```python
from build123d import *

# Parameters (mm, degrees)
SKETCH1_R           = 9
BOSS_EXTRUDE1_DEPTH = 27
BOSS_EXTRUDE2_DEPTH = 11.5


with BuildPart() as part:
    # Sketch1 → Boss-Extrude1 (new body, symmetric)
    with BuildSketch(Plane.XY):
        Circle(SKETCH1_R)
    extrude(amount=BOSS_EXTRUDE1_DEPTH, both=True)

    # Sketch2 → Boss-Extrude2 (add, symmetric)
    with BuildSketch(Plane.XY):
        with BuildLine():
            ThreePointArc((1.592403849, 11.893874473), (0, 12), (-1.592403849, 11.893874473))
            ThreePointArc((-1.592403849, 11.893874473), (-2.170910027, 15.684139908), (-4.926417678, 18.350215499))
            ThreePointArc((-4.926417678, 18.350215499), (-5.35291858, 18.230366499), (-5.776509232, 18.100606097))
            ThreePointArc((-5.776509232, 18.100606097), (-6.653200491, 14.368020679), (-5.090698654, 10.866682438))
            ThreePointArc((-5.090698654, 10.866682438), (-6.487689809, 10.095042394), (-7.769929381, 9.144845401))
            ThreePointArc((-7.769929381, 9.144845401), (-10.305771951, 12.020655535), (-14.065241784, 12.773761136))
            ThreePointArc((-14.065241784, 12.773761136), (-14.359241913, 12.442353945), (-14.645435276, 12.104182152))
            ThreePointArc((-14.645435276, 12.104182152), (-13.364966863, 8.490156404), (-10.157540304, 6.389395509))
            ThreePointArc((-10.157540304, 6.389395509), (-10.915583944, 4.984980156), (-11.480557235, 3.492392528))
            ThreePointArc((-11.480557235, 3.492392528), (-15.168624097, 4.540697964), (-18.738451003, 3.141727868))
            ThreePointArc((-18.738451003, 3.141727868), (-18.806607396, 2.703981927), (-18.864539099, 2.264765898))
            ThreePointArc((-18.864539099, 2.264765898), (-15.833450688, -0.083272541), (-11.999434677, -0.116479348))
            ThreePointArc((-11.999434677, -0.116479348), (-11.877857303, -1.707778059), (-11.546189284, -3.268870296))
            ThreePointArc((-11.546189284, -3.268870296), (-15.215545269, -4.380899128), (-17.462334429, -7.4877818))
            ThreePointArc((-17.462334429, -7.4877818), (-17.283007912, -7.892885247), (-17.094285049, -8.293697527))
            ThreePointArc((-17.094285049, -8.293697527), (-13.274925794, -8.630263043), (-10.031593324, -6.585372836))
            ThreePointArc((-10.031593324, -6.585372836), (-9.068994892, -7.858328807), (-7.945987817, -8.992289898))
            ThreePointArc((-7.945987817, -8.992289898), (-10.431638326, -11.911591701), (-10.642050057, -15.739973653))
            ThreePointArc((-10.642050057, -15.739973653), (-10.272175532, -15.983817124), (-9.896716278, -16.218970587))
            ThreePointArc((-9.896716278, -16.218970587), (-6.501705756, -14.437206007), (-4.87879197, -10.963456978))
            ThreePointArc((-4.87879197, -10.963456978), (-3.380790682, -11.513915683), (-1.822991362, -11.860720994))
            ThreePointArc((-1.822991362, -11.860720994), (-2.335759921, -15.660438072), (-0.442989984, -18.994835084))
            ThreePointArc((-0.442989984, -18.994835084), (0, -19), (0.442989984, -18.994835084))
            ThreePointArc((0.442989984, -18.994835084), (2.335759921, -15.660438072), (1.822991362, -11.860720994))
            ThreePointArc((1.822991362, -11.860720994), (3.380790682, -11.513915683), (4.87879197, -10.963456978))
            ThreePointArc((4.87879197, -10.963456978), (6.501705756, -14.437206007), (9.896716278, -16.218970587))
            ThreePointArc((9.896716278, -16.218970587), (10.272175532, -15.983817124), (10.642050057, -15.739973653))
            ThreePointArc((10.642050057, -15.739973653), (10.431638326, -11.911591701), (7.945987817, -8.992289898))
            ThreePointArc((7.945987817, -8.992289898), (9.068994892, -7.858328807), (10.031593324, -6.585372836))
            ThreePointArc((10.031593324, -6.585372836), (13.274925794, -8.630263043), (17.094285049, -8.293697527))
            ThreePointArc((17.094285049, -8.293697527), (17.283007912, -7.892885247), (17.462334429, -7.4877818))
            ThreePointArc((17.462334429, -7.4877818), (15.215545269, -4.380899128), (11.546189284, -3.268870296))
            ThreePointArc((11.546189284, -3.268870296), (11.877857303, -1.707778059), (11.999434677, -0.116479348))
            ThreePointArc((11.999434677, -0.116479348), (15.833450688, -0.083272541), (18.864539099, 2.264765898))
            ThreePointArc((18.864539099, 2.264765898), (18.806607396, 2.703981927), (18.738451003, 3.141727868))
            ThreePointArc((18.738451003, 3.141727868), (15.168624097, 4.540697964), (11.480557235, 3.492392528))
            ThreePointArc((11.480557235, 3.492392528), (10.915583944, 4.984980156), (10.157540304, 6.389395509))
            ThreePointArc((10.157540304, 6.389395509), (13.364966863, 8.490156404), (14.645435276, 12.104182152))
            ThreePointArc((14.645435276, 12.104182152), (14.359241913, 12.442353945), (14.065241784, 12.773761136))
            ThreePointArc((14.065241784, 12.773761136), (10.305771951, 12.020655535), (7.769929381, 9.144845401))
            ThreePointArc((7.769929381, 9.144845401), (6.487689809, 10.095042394), (5.090698654, 10.866682438))
            ThreePointArc((5.090698654, 10.866682438), (6.653200491, 14.368020679), (5.776509232, 18.100606097))
            ThreePointArc((5.776509232, 18.100606097), (5.35291858, 18.230366499), (4.926417678, 18.350215499))
            ThreePointArc((4.926417678, 18.350215499), (2.170910027, 15.684139908), (1.592403849, 11.893874473))
        make_face()
    extrude(amount=BOSS_EXTRUDE2_DEPTH, both=True)


solid = part.part
```
Geometry: final body of the model. Coordinates: model frame, mm. A direction names the side the tool comes from. Coordinates: 2 decimals unless noted, no trailing zeros. Order: outer loops, then holes, each group sorted by start corner. A loop starts at its lowest first (then second) coordinate and runs counter-clockwise, first axis right, second up. Notation, with made-up numbers: (-20.75, -26) -> (31.25, -26) arc R18 ccw to (31.25, -19) -> close; hole circle Ø8 at (-35, -27.5). An arc over 180 degrees is marked (long way). Write each question's results on one line, items separated by ' | '. Start each with the question number.
1) Material intervals for line 1 along X through (y, z) = (10.5, -9); line 2 along Z through (x, y) = (9.5, -12.5); line 3 along X through (y, z) = (-15.5, -2), sorted ascending.
2) Cut plane A-A, the plane y = -14.5. Output: boundary loops of the cut face in (x, z), and give its area (3 significant figures).
3) Cut plane B-B, the plane y = 7. Output: boundary loops of the cut face in (x, z), and give its area (3 significant figures).
4) Set-up query: faces 1 (the flat face through (0, 0, -27)), 2 (the flat face through (-4.5, 8.2, 11.5)). Return all of +Z, -Z, +X, -X, +Y, -Y with unobstructed straight access to the full face (end or side cutting, diameter ignored); none if empty.
5) First-contact query: pin 1 (6 mm diameter, centred on y = 13.5, z = -20.5, fed in from -X); pin 2 (3 mm diameter, centred on x = 2.5, z = -8, fed in from -Y); pin 3 (4 mm diameter, centred on y = 9.5, z = -21.5, fed in from +X); pin 4 (6 mm diameter, centred on x = -10, z = -4, fed in from -Y). Flat tips, straight axial feed; report the tip coordinate or a pass-through.
6) Mould query, pull axis Y, two halves, no side actions, for faces 3 (the flat face through (-4.5, 8.2, -11.5)), 4 (the cylindrical face through (-10.906, 5.005, 0.161)). Classes: released by +Y, released by -Y, zero draft, split by the parting line, or undercut.
Checks:
1) line 1: -14.4 to -8.56, -5.81 to 5.81, 8.56 to 14.4 | line 2: -11.5 to 11.5 | line 3: -10.7 to -7.86, -2.36 to 2.36, 7.86 to 10.7
2) outline: (-10.85, -11.5) -> (-6.56, -11.5) -> (-6.56, 11.5) -> (-10.85, 11.5) -> close; (-2.44, -11.5) -> (2.44, -11.5) -> (2.44, 11.5) -> (-2.44, 11.5) -> close; (6.56, -11.5) -> (10.85, -11.5) -> (10.85, 11.5) -> (6.56, 11.5) -> close | area: 310 mm^2
3) outline: (-11.65, -11.5) -> (-5.66, -11.5) -> (-5.66, -27) -> (5.66, -27) -> (5.66, -11.5) -> (11.65, -11.5) -> (11.65, 11.5) -> (5.66, 11.5) -> (5.66, 27) -> (-5.66, 27) -> (-5.66, 11.5) -> (-11.65, 11.5) -> close | area: 886 mm^2
4) face 1: -Z, +X, -X, +Y, -Y | face 2: +Z
5) pin 1: through | pin 2: y = -18.43 | pin 3: x = 4.97 | pin 4: y = -16.22
6) face 3: zero draft | face 4: undercut
